from build123d import *

# Parameters (mm, degrees)
SKETCH1_R           = 6.858
BOSS_EXTRUDE1_DEPTH = 18.2118
SKETCH2_R           = 0.635
BOSS_EXTRUDE2_DEPTH = 4.191


with BuildPart() as part:
    # Sketch1 → Boss-Extrude1 (new body)
    with BuildSketch(Plane.XY):
        Circle(SKETCH1_R)
    extrude(amount=BOSS_EXTRUDE1_DEPTH)

    # Sketch2 → Boss-Extrude2 (add)
    with BuildSketch(Plane.XY.offset(18.2118)):
        with BuildLine():
            Line((-7.4676, 7.4676), (7.4676, 7.4676))
            Line((7.4676, 7.4676), (7.4676, 2.0828))
            Line((7.4676, 2.0828), (8.9154, 2.0828))
            ThreePointArc((8.9154, 2.0828), (10.9474, 0.0508), (8.9154, -1.9812))
            Line((8.9154, -1.9812), (7.4676, -1.9812))
            Line((7.4676, -1.9812), (7.4676, -7.4676))
            Line((7.4676, -7.4676), (-7.4676, -7.4676))
            Line((-7.4676, -7.4676), (-7.4676, -1.9812))
            Line((-7.4676, -1.9812), (-8.9154, -1.9812))
            ThreePointArc((-8.9154, -1.9812), (-10.9474, 0.0508), (-8.9154, 2.0828))
            Line((-8.9154, 2.0828), (-7.4676, 2.0828))
            Line((-7.4676, 2.0828), (-7.4676, 7.4676))
        make_face()
        with Locations((-8.9154, 0.0508)):
            Circle(SKETCH2_R, mode=Mode.SUBTRACT)
        with Locations((8.9154, 0.0508)):
            Circle(SKETCH2_R, mode=Mode.SUBTRACT)
    extrude(amount=BOSS_EXTRUDE2_DEPTH)


solid = part.part
Work out the finished part from the listing and answer in its coordinate system (mm). A direction names the side the tool comes from. Round coordinates to 2 decimals unless told otherwise and drop trailing zeros. Write each loop counter-clockwise with the first axis right and the second up, starting at its lowest first coordinate (ties: lowest second). Pieces come first, ordered by that corner, then holes. Notation, with made-up numbers: (-28.5, 48.5) -> (23.5, 48.5) arc R19 ccw to (23.5, 75.5) -> close; hole circle Ø8 at (-13.5, 12). An arc over 180 degrees is marked (long way). Answer as CSV lines item,"result". Start each with the question number.
(1) The part is cut by section C-C, the plane z = 17.25. Give the vertices of the cut face in (x, y).
(2) The part is cut by section B-B, the plane y = 2.75. Give the vertices of the cut face in (x, z), then the cut area to 3 significant figures.
(3) A tool of negligible diameter and unlimited length cuts with its end or side. For faces 1 (the flat face through (5, 5, 18.212)), 2 (the flat face through (8, -1.981, 20)), 3 (the flat face through (8, 2.083, 20)), from which of +Z, -Z, +X, -X, +Y, -Y can it reach the whole face along a straight path? Write none if from no direction.
(4) Find the intervals of material crossed by probe 1 along Z at (x, y) = (-5, 6.25); probe 2 along Y at (x, z) = (0, 14.75); probe 3 along X at (y, z) = (-4, 19.75), in increasing order.
(5) Each of these flat-tipped pins is pushed along its axis until it touches: pin 1 (2 mm diameter, centred on y = -5, z = 14.5, fed in from +X); pin 2 (2 mm diameter, centred on y = -4, z = 19.5, fed in from +X); pin 3 (0.7 mm diameter, centred on x = 8.5, z = 20.5, fed in from -Y). Where does it stop, or does it pass through?
(6) The part is cut by section A-A, the plane x = 0. Give the vertices of the cut face in (y, z).
(7) The mould has two halves that part along X. Classify faces 4 (the cylindrical face through (8.28, 0.08, 20.28)), 5 (the flat face through (0, 0, 22.403)), 6 (the flat face through (7.468, 5, 20)): +X half, -X half, draft (parallel to the pull), parting line (faces both ways), or undercut.
Output values:
1,outline,"circle Ø13.72 at (0, 0)"
2,outline,"(-7.47, 18.21) -> (-6.28, 18.21) -> (-6.28, 0) -> (6.28, 0) -> (6.28, 18.21) -> (7.47, 18.21) -> (7.47, 22.4) -> (-7.47, 22.4) -> close"
2,area,"291 mm²"
3,face 1,"-Z"
3,face 2,"+Z, -Z, +X, -Y"
3,face 3,"+Z, -Z, +X, +Y"
4,probe 1,"z = 18.21 to 22.4"
4,probe 2,"y = -6.86 to 6.86"
4,probe 3,"x = -7.47 to 7.47"
5,pin 1,"stops at x = 5.57"
5,pin 2,"stops at x = 7.47"
5,pin 3,"stops at y = -1.98"
6,outline,"(-7.47, 18.21) -> (-6.86, 18.21) -> (-6.86, 0) -> (6.86, 0) -> (6.86, 18.21) -> (7.47, 18.21) -> (7.47, 22.4) -> (-7.47, 22.4) -> close"
7,face 4,"undercut"
7,face 5,"draft"
7,face 6,"+X half"
